Autodesk Inventor part; units mm, degrees
ref_plane "YZ Plane" through (0, 0, 0) normal (1, 0, 0) x (0, 1, 0)
ref_plane "XZ Plane" through (0, 0, 0) normal (0, 1, 0) x (-1, 0, 0)
ref_plane "XY Plane" through (0, 0, 0) normal (0, 0, 1) x (1, 0, 0)
sketch "Boceto1" plane through (0, 0, 0) normal (0, 1, 0) x (-1, 0, 0)
  line L0 (-5.4361, 12.1513) -> (1.0639, 12.1513)
  line L1 (1.0639, 12.1513) -> (1.0639, -17.8487)
  line L2 (1.0639, -17.8487) -> (-5.4361, -17.8487)
  line L3 (-5.4361, -17.8487) -> (-5.4361, -18.8487)
  line L4 (-5.4361, -18.8487) -> (2.0639, -18.8487)
  line L5 (2.0639, -18.8487) -> (2.0639, 13.1513)
  line L6 (2.0639, 13.1513) -> (-5.4361, 13.1513)
  line L7 (-5.4361, 13.1513) -> (-5.4361, 12.1513)
  point P0 (0, 0)
  point P1 (0, 0)
  dimension "d0" = 6.5
  dimension "d1" = 30
  dimension "d2" = 1
  dimension "d3" = 7.5
  dimension "d4" = 32
extrude "Extrusión1" add sketch "Boceto1" along normal blind 148
properties part number "Tapa cable canal 150mm"
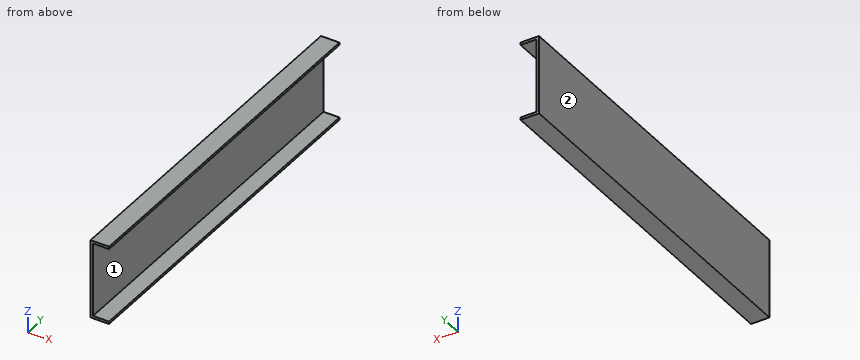
Verification items for the finished model (mm, model axes). Face numbers are marked on the shaded views. A direction names the side the tool comes from. Give positions to 0.01 mm unless a question says otherwise; leave off trailing zeros. Write each loop counter-clockwise with the first axis right and the second up, starting at its lowest first coordinate (ties: lowest second). Pieces come first, ordered by that corner, then holes. Notation, with made-up numbers: M 68.25,-28 L 126.25,-28 A21 cw 126.25,-2 Z; hole C 86.5,71.5 d6. An arc over 180 degrees is marked long. Use CSV: the item, a comma, the result in double quotes.
1) Material ranges on line 1 along Z through (x, y) = (-0.5, 119.5); line 2 along X through (y, z) = (115.5, -16), recorded low to high.
Final values:
line 1,"-18.85 to -17.85, 12.15 to 13.15"
line 2,"-2.06 to -1.06"
2) Cross-section at C-C (z = -13). Enter the section's corners in (x, y), plus the area to 3 significant figures.
Final values:
outline,"M -2.06,0 L -1.06,0 L -1.06,148 L -2.06,148 Z"
area,"148 mm²"
3) Access from +Z, -Z, +X, -X, +Y, -Y to the whole of each face (thin tool, end or side, straight path). Record for the marked faces 1 and 2.
Final values:
face 1,"+X, +Y, -Y"
face 2,"+Z, -Z, -X, +Y, -Y"
4) Go/stop test with a flat-tipped pin: pin 1 Ø2 at (y, z) = (66, 7.5) entering from +X. Record where the tip stops, or that it passes through.
Final values:
pin 1,"x = -1.06"
5) Cross-section at A-A (x = 3.5). Enter the section's corners in (y, z).
Final values:
outline,"M 0,-18.85 L 148,-18.85 L 148,-17.85 L 0,-17.85 Z; M 0,12.15 L 148,12.15 L 148,13.15 L 0,13.15 Z"
6) Cross-section at B-B (y = 39.5). Enter the section's corners in (x, z), plus the area to 3 significant figures.
Final values:
outline,"M -2.06,-18.85 L 5.44,-18.85 L 5.44,-17.85 L -1.06,-17.85 L -1.06,12.15 L 5.44,12.15 L 5.44,13.15 L -2.06,13.15 Z"
area,"45.0 mm²"
